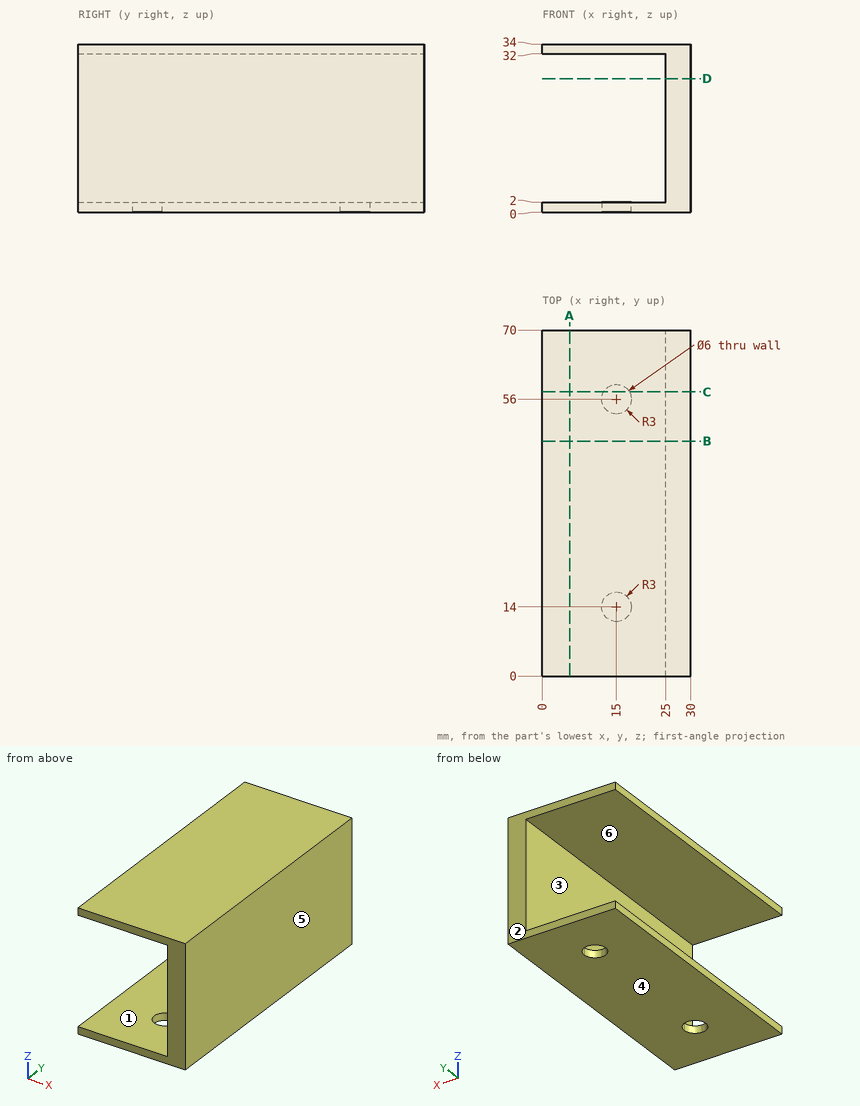
Print and shaded views of the part. All mm, measured from the part's lowest x, y and z. A direction names the side the tool comes from. Coordinates: 2 decimals unless noted, no trailing zeros. Order: outer loops, then holes, each group sorted by start corner. A loop starts at its lowest first (then second) coordinate and runs counter-clockwise, first axis right, second up. Notation, with made-up numbers: (76.25, -5) -> (117.25, -5) arc R18 ccw to (117.25, 28) -> close; hole circle Ø6 at (-37.5, -30.75). An arc over 180 degrees is marked (long way). Use one line per item in the form item = value. Start each with the question number.
1) Band-saw the part on C-C on y = 57.5. Give the cut face in (x, z).
2) Band-saw the part on B-B on y = 47.5. Give the cut face in (x, z), then the cut area to 3 significant figures.
3) Band-saw the part on A-A on x = 5.5. Give the cut face in (y, z), then the cut area to 3 significant figures.
4) Drill centre lines: L1, parallel to Y at x = 15, z = 0.6; L2, parallel to Z at x = 3, y = 34; L3, parallel to X at y = 56, z = 1. Where is each one in solid material? Low to high. Write a range as [from, to].
5) Drop a flat-ended pin along its axis: pin 1 (12 mm diameter, centred on y = 60, z = 24, fed in from -X). Give the stop position or say it passes through.
6) Tool access for the marked faces 5 and 6: list every direction of +Z, -Z, +X, -X, +Y, -Y with a clear straight run to the whole face (end or side of a thin tool).
7) Band-saw the part on D-D on z = 27. Give the cut face in (x, y).
8) Pull direction Z, two halves, no side cores. Call the marked faces 1, 2, 3 and 4: +Z half, -Z half, draft (parallel to the pull), parting line (faces both ways), or undercut.
Entries:
q1.outline = (0, 0) -> (12.4, 0) -> (12.4, 2) -> (0, 2) -> close; (0, 32) -> (25, 32) -> (25, 2) -> (17.6, 2) -> (17.6, 0) -> (30, 0) -> (30, 34) -> (0, 34) -> close
q2.outline = (0, 0) -> (30, 0) -> (30, 34) -> (0, 34) -> (0, 32) -> (25, 32) -> (25, 2) -> (0, 2) -> close
q2.area = 270 mm2
q3.outline = (0, 0) -> (70, 0) -> (70, 2) -> (0, 2) -> close; (0, 32) -> (70, 32) -> (70, 34) -> (0, 34) -> close
q3.area = 280 mm2
q4.L1 = [0, 11], [17, 53], [59, 70]
q4.L2 = [0, 2], [32, 34]
q4.L3 = [0, 12], [18, 30]
q5.pin_1 = 25
q6.face_5 = +Z, -Z, +X, +Y, -Y
q6.face_6 = -X, +Y, -Y
q7.outline = (25, 0) -> (30, 0) -> (30, 70) -> (25, 70) -> close
q8.face_1 = undercut
q8.face_2 = draft
q8.face_3 = undercut
q8.face_4 = -Z half
